```python
from build123d import *

# Parameters (mm, degrees)
SKETCH_1_R                  = 4.95
EXTRUDE_1_DEPTH             = 20.44
SKETCH_2_W                  = 7.000357134
SKETCH_2_H                  = 7.000357134
EXTRUDE_2_DEPTH             = 5.1
EXTRUDE_3_DEPTH             = 2
EXTRUDE_3_DEPTH_BACK        = 9.000357
EXTRUDE_4_DEPTH             = 82.4
EXTRUDE_4_DIRECTION_2_REACH = 24.791
FILLET_1_R                  = 2


with BuildPart() as part:
    # 草图1 → 凸台-拉伸1 (new body)
    with BuildSketch(Plane.XY):
        Circle(SKETCH_1_R)
    extrude(amount=-EXTRUDE_1_DEPTH)

    # 草图2 → 凸台-拉伸2 (add)
    with BuildSketch(Plane.XY):
        Rectangle(SKETCH_2_W, SKETCH_2_H)
    extrude(amount=EXTRUDE_2_DEPTH)

    # 草图3 → 凸台-拉伸3 (add, two sides: drawn at the far end of the back side and taken through both)
    with BuildSketch(Plane.XZ.offset(3.500178567).offset(-EXTRUDE_3_DEPTH_BACK)):
        with BuildLine():
            ThreePointArc((0.5, 5.1), (0, 5.6), (-0.5, 5.1))
            Line((-0.5, 5.1), (0.5, 5.1))
        make_face()
        with BuildLine():
            Line((0.5, 5.1), (-0.5, 5.1))
            ThreePointArc((-0.5, 5.1), (0, 4.6), (0.5, 5.1))
        make_face()
        with BuildLine():
            ThreePointArc((0.5, 5.1), (0, 5.6), (-0.5, 5.1))
            Line((-0.5, 5.1), (0.5, 5.1))
        make_face()
        with BuildLine():
            Line((0.5, 5.1), (-0.5, 5.1))
            ThreePointArc((-0.5, 5.1), (0, 4.6), (0.5, 5.1))
        make_face()
    extrude(amount=EXTRUDE_3_DEPTH + EXTRUDE_3_DEPTH_BACK)

    # 草图5 → 凸台-拉伸4 (add)
    with BuildSketch(Plane.ZY.offset(3.500178567)):
        with BuildLine():
            ThreePointArc((9.835, 0), (7.013225527, 4.331257679), (1.911116967, 3.500178567))
            Line((1.911116967, 3.500178567), (5.1, 3.500178567))
            Line((5.1, 3.500178567), (5.1, -3.500178567))
            Line((5.1, -3.500178567), (1.911116967, -3.500178567))
            ThreePointArc((1.911116967, -3.500178567), (7.013225527, -4.331257679), (9.835, 0))
        make_face()
        with BuildLine():
            Line((5.1, 3.500178567), (1.911116967, 3.500178567))
            ThreePointArc((1.911116967, 3.500178567), (0.365, 0), (1.911116967, -3.500178567))
            Line((1.911116967, -3.500178567), (5.1, -3.500178567))
            Line((5.1, -3.500178567), (5.1, 3.500178567))
        make_face()
        with BuildLine():
            ThreePointArc((9.835, 0), (7.013225527, 4.331257679), (1.911116967, 3.500178567))
            Line((1.911116967, 3.500178567), (5.1, 3.500178567))
            Line((5.1, 3.500178567), (5.1, -3.500178567))
            Line((5.1, -3.500178567), (1.911116967, -3.500178567))
            ThreePointArc((1.911116967, -3.500178567), (7.013225527, -4.331257679), (9.835, 0))
        make_face()
        with BuildLine():
            Line((5.1, 3.500178567), (1.911116967, 3.500178567))
            ThreePointArc((1.911116967, 3.500178567), (0.365, 0), (1.911116967, -3.500178567))
            Line((1.911116967, -3.500178567), (5.1, -3.500178567))
            Line((5.1, -3.500178567), (5.1, 3.500178567))
        make_face()
    extrude(amount=EXTRUDE_4_DEPTH)

    # 凸台-拉伸4 direction 2: up to this face of the body (flat: up to its plane)
    extrude_4_direction_2_end = Plane(part.part.faces().sort_by_distance((3.500178567, 0, 2.55))[0])
    # 草图5 → 凸台-拉伸4 direction 2 (add, up to the picked face)
    with BuildSketch(Plane.ZY.offset(3.500178567), mode=Mode.PRIVATE) as extrude_4_direction_2_sk1:
        with BuildLine():
            ThreePointArc((9.835, 0), (7.013225527, 4.331257679), (1.911116967, 3.500178567))
            Line((1.911116967, 3.500178567), (5.1, 3.500178567))
            Line((5.1, 3.500178567), (5.1, -3.500178567))
            Line((5.1, -3.500178567), (1.911116967, -3.500178567))
            ThreePointArc((1.911116967, -3.500178567), (7.013225527, -4.331257679), (9.835, 0))
        make_face()
    extrude_4_direction_2_tool1 = split(extrude(extrude_4_direction_2_sk1.sketch, amount=-EXTRUDE_4_DIRECTION_2_REACH, mode=Mode.PRIVATE), bisect_by=extrude_4_direction_2_end, keep=Keep.BOTH, mode=Mode.PRIVATE)
    # 草图5 → 凸台-拉伸4 direction 2 (add, up to the picked face)
    with BuildSketch(Plane.ZY.offset(3.500178567), mode=Mode.PRIVATE) as extrude_4_direction_2_sk2:
        with BuildLine():
            Line((5.1, 3.500178567), (1.911116967, 3.500178567))
            ThreePointArc((1.911116967, 3.500178567), (0.365, 0), (1.911116967, -3.500178567))
            Line((1.911116967, -3.500178567), (5.1, -3.500178567))
            Line((5.1, -3.500178567), (5.1, 3.500178567))
        make_face()
    extrude_4_direction_2_tool2 = split(extrude(extrude_4_direction_2_sk2.sketch, amount=-EXTRUDE_4_DIRECTION_2_REACH, mode=Mode.PRIVATE), bisect_by=extrude_4_direction_2_end, keep=Keep.BOTH, mode=Mode.PRIVATE)
    # 草图5 → 凸台-拉伸4 direction 2 (add, up to the picked face)
    with BuildSketch(Plane.ZY.offset(3.500178567), mode=Mode.PRIVATE) as extrude_4_direction_2_sk3:
        with BuildLine():
            ThreePointArc((9.835, 0), (7.013225527, 4.331257679), (1.911116967, 3.500178567))
            Line((1.911116967, 3.500178567), (5.1, 3.500178567))
            Line((5.1, 3.500178567), (5.1, -3.500178567))
            Line((5.1, -3.500178567), (1.911116967, -3.500178567))
            ThreePointArc((1.911116967, -3.500178567), (7.013225527, -4.331257679), (9.835, 0))
        make_face()
    extrude_4_direction_2_tool3 = split(extrude(extrude_4_direction_2_sk3.sketch, amount=-EXTRUDE_4_DIRECTION_2_REACH, mode=Mode.PRIVATE), bisect_by=extrude_4_direction_2_end, keep=Keep.BOTH, mode=Mode.PRIVATE)
    # 草图5 → 凸台-拉伸4 direction 2 (add, up to the picked face)
    with BuildSketch(Plane.ZY.offset(3.500178567), mode=Mode.PRIVATE) as extrude_4_direction_2_sk4:
        with BuildLine():
            Line((5.1, 3.500178567), (1.911116967, 3.500178567))
            ThreePointArc((1.911116967, 3.500178567), (0.365, 0), (1.911116967, -3.500178567))
            Line((1.911116967, -3.500178567), (5.1, -3.500178567))
            Line((5.1, -3.500178567), (5.1, 3.500178567))
        make_face()
    extrude_4_direction_2_tool4 = split(extrude(extrude_4_direction_2_sk4.sketch, amount=-EXTRUDE_4_DIRECTION_2_REACH, mode=Mode.PRIVATE), bisect_by=extrude_4_direction_2_end, keep=Keep.BOTH, mode=Mode.PRIVATE)
    add(extrude_4_direction_2_tool1.solids().sort_by(Axis((-3.500179, 0, 6.679951), (1, 0, 0)))[0])
    add(extrude_4_direction_2_tool2.solids().sort_by(Axis((-3.500179, 0, 2.947224), (1, 0, 0)))[0])
    add(extrude_4_direction_2_tool3.solids().sort_by(Axis((-3.500179, 0, 6.679951), (1, 0, 0)))[0])
    add(extrude_4_direction_2_tool4.solids().sort_by(Axis((-3.500179, 0, 2.947224), (1, 0, 0)))[0])

    # 圆角1
    fillet_1_edges = [part.edges().sort_by_distance(p)[0] for p in [
        (-85.900178567, -3.500178567, 8.288883033),
    ]]
    fillet(fillet_1_edges, radius=FILLET_1_R)


solid = part.part
```
Geometry: final body of the model. Coordinates: model frame, mm. A direction names the side the tool comes from. Coordinates: 2 decimals unless noted, no trailing zeros. Order: outer loops, then holes, each group sorted by start corner. A loop starts at its lowest first (then second) coordinate and runs counter-clockwise, first axis right, second up. Notation, with made-up numbers: (72.25, -21) -> (94.25, -21) arc R27 cw to (94.25, 18) -> close; hole circle Ø2 at (20, -33.75). An arc over 180 degrees is marked (long way). Answer in a Markdown table with one row per item.
Item 1: Section A-A on x = -45.5. Output: boundary loops of the cut face in (y, z) (3 decimals), plus the area to 3 significant figures.
Return value:
| item | result |
|---|---|
| outline | circle Ø9.47 at (0, 5.1) |
| area | 70.4 mm² |
Item 2: Contact query for flat-ended pins moving along their axis: P1, Ø0.7, axis at x = 0, y = 4.5, coming from the +Z side; P2, Ø3, axis at y = -1, z = 3.5, coming from the +X side; P3, Ø0.6, axis at y = 1.5, z = 1.5, coming from the -X side. Output: stop coordinate, or through.
Return value:
| item | result |
|---|---|
| P1 | stops at z = 7.38 |
| P2 | stops at x = 3.5 |
| P3 | stops at x = -85.7 |
Item 3: Section B-B on z = -13. Output: boundary loops of the cut face in (x, y), plus the area to 3 significant figures.
Return value:
| item | result |
|---|---|
| outline | circle Ø9.9 at (0, 0) |
| area | 77.0 mm² |
Item 4: Access query for faces 1 (the flat face through (3.5, 0, 5)), 2 (the flat face through (0, -4, 0)), 3 (the flat face through (0, 3.5, 1)), 4 (the flat face through (-85.9, 0, 5)), 5 (the flat face through (0, 0, -20.44)). Directions: +Z, -Z, +X, -X, +Y, -Y. A direction counts if a zero-diameter tool reaches every point of the face in a straight line with its end or side. Return the directions, or none.
Return value:
| item | result |
|---|---|
| face 1 | +Z, +X, +Y, -Y |
| face 2 | +X, -X, -Y |
| face 3 | +X, -X, +Y |
| face 4 | +Z, -Z, -X, +Y, -Y |
| face 5 | -Z, +X, -X, +Y, -Y |
Item 5: Draft query along Z for faces 6 (the cylindrical face through (4.72, 1.49, -10.08)), 7 (the flat face through (4, 0, 0)), 8 (the flat face through (-4, 0, 0)). Return one class per face: released by +Z, released by -Z, zero draft, split by the parting line, or undercut.
Return value:
| item | result |
|---|---|
| face 6 | zero draft |
| face 7 | released by +Z |
| face 8 | undercut |
Item 6: Ray query, L1, parallel to Y at x = -80, z = 4.5; L2, parallel to Z at x = -50, y = 0.25; L3, parallel to X at y = 0.75, z = 5. Return the intervals inside material, ascending.
Return value:
| item | result |
|---|---|
| L1 | y = -4.7 to 4.7 |
| L2 | z = 0.37 to 9.83 |
| L3 | x = -85.9 to 3.5 |
